Input: part model. Units: mm. Frame: model coordinates. Face numbers are marked on the shaded views. Coordinates: 2 decimals unless noted, no trailing zeros. Order: outer loops, then holes, each group sorted by start corner. A loop starts at its lowest first (then second) coordinate and runs counter-clockwise, first axis right, second up. Notation, with made-up numbers: M 23.5,40 L 36.5,40 A16 cw 36.5,62 Z; hole C -39,85 d11. An arc over 180 degrees is marked long. Answer in a Markdown table with one row per item.
Autodesk Inventor part; units mm, degrees
ref_plane "Work Plane1" through (29, 0, 0) normal (0, -1, 0) x (1, 0, 0)
ref_plane "YZ Plane" through (0, 0, 0) normal (1, 0, 0) x (0, 1, 0)
ref_plane "XZ Plane" through (0, 0, 0) normal (0, 1, 0) x (-1, 0, 0)
sketch "Sketch1" plane through (0, 0, 0) normal (0, 0, 1) x (1, 0, 0)
  line L0 (-1.7103, 0) -> (44.45, 0)
  line L1 (44.45, 0) -> (44.45, 3.175)
  line L2 (44.45, 3.175) -> (12.7, 3.175)
  line L3 (12.7, 3.175) -> (9.5249, 3.175)
  line L4 (9.5249, 3.175) -> (0, 3.175)
  line L5 (0, 3.175) -> (0, 4.7625)
  line L6 (0, 4.7625) -> (-6.35, 4.7625)
  line L7 (-6.35, 4.7625) -> (-6.35, 2.757)
  line L8 (-6.35, 2.757) -> (-3.302, 2.757)
  line L9 (-3.302, 2.757) -> (-1.7103, 0)
  line L10 (-16.51, 0) -> (54.61, 0)
  line L11 (0, -0.9525) -> (0, 5.715)
  line L12 (12.7, 3.175) -> (0, 3.175) construction
  dimension "d1" = 31.75
  dimension "d2" = 3.1751
  dimension "d3" = 6.35
  dimension "d4" = 3.048
  dimension "d5" = 60
  dimension "d6" = 6.35
  dimension "d7" = 6.35
  dimension "d8" = 5.5139
  dimension "d9" = 9.525
  dimension "d26" = 44.45
revolve "Body" add sketch "Sketch1" angle 360 about axis through (-1.7103, 0, 0) along (1, 0, 0)
sketch "Sketch2" plane through (-6.35, 0, 0) normal (-1, 0, 0) x (0, 0, 1)
  circle A0 centre (0, 0) radius 2.757
  line L0 (0, -6.6675) -> (0, 6.6675)
  line L1 (-6.6675, 0) -> (6.6675, 0)
  line L2 (2.757, 0) -> (1.3785, -2.3876)
  line L3 (1.3785, -2.3876) -> (-1.3785, -2.3876)
  line L4 (-1.3785, -2.3876) -> (-2.757, 0)
  line L5 (-2.757, 0) -> (-1.3785, 2.3876)
  line L6 (-1.3785, 2.3876) -> (1.3785, 2.3876)
  line L7 (1.3785, 2.3876) -> (2.757, 0)
extrude "Slot" add sketch "Sketch2" against normal up to next contours L7 A0 | A0 L2 | L6 L0 A0 | A0 L0 L3 | L0 L6 A0 | A0 L3 L0 | L4 A0 | A0 L5
fillet "Fillet1" radius 0.635 1 edges at (-6.35, -4.7625, 0)
thread "Thread"
chamfer "Chamfer1" distance 0.7556 distance2 0.7556 1 edges at (44.45, -3.175, 0) measured on face at (44.45, 0.6012, -0.3644)
ref_plane "Work Plane1" through (29, 0, 0) normal (0, -1, 0) x (1, 0, 0)
equation "\"d17\" = RR"
equation "\"d13\" = GEL"
equation "\"d15\" = -0.5 * SPD + 0.5 * GD"
equation "\"d16\" = GUL"
equation "\"d1\" = GEL"
equation "\"d3\" = KOH"
equation "\"d4\" = INTI"
equation "\"d6\" = GD"
equation "\"d7\" = BDM"
equation "\"d8\" = 1.1547 * SW"
equation "\"d9\" = KOD"
equation "\"d26\" = NLG"
equation "\"GD\" = 6.35"
equation "\"NLG\" = 44.45"
equation "\"GEL\" = 31.75"
equation "\"KOD\" = 9.525"
equation "\"KOH\" = 6.35"
equation "\"INTI\" = 3.048"
equation "\"GAL\" = 3.175"
equation "\"GUL\" = 0.75565"
equation "\"BDM\" = 6.35"
equation "\"SW\" = 4.7752"
equation "\"RR\" = 0.635"
equation "\"SPD\" = 4.8387"
equation "\"R\" = 0.1778"
equation "\"PHH\" = 0.2032"
equation "\"GD1\" = SPD"
equation "\"THREADDIA\" = 6.35"
equation "\"FAWI\" = 45deg"
equation "\"KOH1\" = 5.715"
equation "\"NND\" = 6.35"
equation "\"TOA\" = 30deg"
equation "\"E0\" = 1.155 * SW"
properties part number "am-1058" material "Steel"
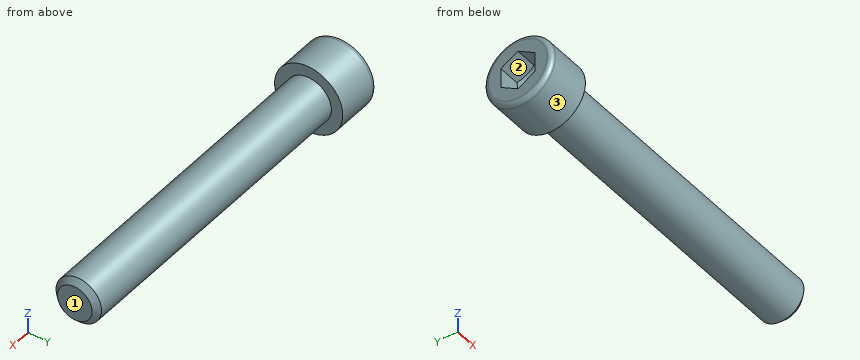
1) Cut plane A-A, the plane x = 6.5. Output: boundary loops of the cut face in (y, z) (3 decimals).
Resolved:
| item | result |
|---|---|
| outline | C 0,0 d6.35 |
2) Material intervals for probe 1 along Z at (x, y) = (38.5, -0.25); probe 2 along X at (y, z) = (-3, -2.25), sorted ascending.
Resolved:
| item | result |
|---|---|
| probe 1 | z = -3.17 to 3.17 |
| probe 2 | x = -6.35 to 0 |
3) Contact query for flat-ended pins moving along their axis: pin 1 (1 mm diameter, centred on x = 6.5, z = 3, fed in from +Y); pin 2 (1.5 mm diameter, centred on x = 20.5, y = -1.5, fed in from -Z); pin 3 (5 mm diameter, centred on x = 31, y = -0.5, fed in from +Z) (3 decimals); pin 4 (0.8 mm diameter, centred on x = -4.5, z = 0.5, fed in from +Y). Output: stop coordinate, or through.
Resolved:
| item | result |
|---|---|
| pin 1 | stops at y = 1.96 |
| pin 2 | stops at z = -3.09 |
| pin 3 | stops at z = 3.175 |
| pin 4 | stops at y = 4.76 |
4) Mould query, pull axis Y, two halves, no side actions, for the marked faces 1, 2 and 3. Classes: +Y half, -Y half, draft (parallel to the pull), parting line (faces both ways), or undercut.
Resolved:
| item | result |
|---|---|
| face 1 | draft |
| face 2 | undercut |
| face 3 | parting line |
